Geometry check sheet. Reference: the model listing, model coordinates, mm. A direction names the side the tool comes from. Round coordinates to 2 decimals unless told otherwise and drop trailing zeros. Order: outer loops, then holes, each group sorted by start corner. A loop starts at its lowest first (then second) coordinate and runs counter-clockwise, first axis right, second up. Notation, with made-up numbers: (-20.75, 57.25) -> (34.25, 57.25) arc R13 cw to (34.25, 73.25) -> close; hole circle Ø8 at (2, 12.25). An arc over 180 degrees is marked (long way). Answer as a JSON object with one key per item and string values. Group by question number.
from build123d import *

# Parameters (mm, degrees)
ESBO_O1_R                = 3.05
RESSALTO_EXTRUS_O1_DEPTH = 3
ESBO_O2_W                = 22
ESBO_O2_H                = 82.35
RESSALTO_EXTRUS_O2_DEPTH = 3
RESSALTO_EXTRUS_O3_START = 3
RESSALTO_EXTRUS_O3_DEPTH = 3
ESBO_O6_W                = 85.35
ESBO_O6_H                = 6
RESSALTO_EXTRUS_O5_DEPTH = 3
ESBO_O7_R                = 2.75
RESSALTO_EXTRUS_O6_DEPTH = 0.6


with BuildPart() as part:
    # Esboço1 → Ressalto-extrusão1 (new body)
    with BuildSketch(Plane.XY):
        with BuildLine():
            Line((11, -1.428145739), (11, 25.071854261))
            Line((11, 25.071854261), (-11, 25.071854261))
            Line((-11, 25.071854261), (-11, -1.428145739))
            ThreePointArc((-11, -1.428145739), (0, -12.428145739), (11, -1.428145739))
        make_face()
        with Locations((0, -1.428145739)):
            Circle(ESBO_O1_R, mode=Mode.SUBTRACT)
    extrude(amount=-RESSALTO_EXTRUS_O1_DEPTH)

    # Esboço2 → Ressalto-extrusão2 (add)
    with BuildSketch(Plane(origin=(0, 25.071854261, 0), x_dir=(1, 0, 0), z_dir=(0, 1, 0))):
        with Locations((0, -38.175)):
            Rectangle(ESBO_O2_W, ESBO_O2_H)
    extrude(amount=RESSALTO_EXTRUS_O2_DEPTH)

    # Esboço3 → Ressalto-extrusão3 (add)
    with BuildSketch(Plane.XY.offset(79.35).offset(RESSALTO_EXTRUS_O3_START)):
        with BuildLine():
            Line((11, 28.071854261), (-11, 28.071854261))
            Line((-11, 28.071854261), (-11, -1.428145739))
            ThreePointArc((-11, -1.428145739), (0, -12.428145739), (11, -1.428145739))
            Line((11, -1.428145739), (11, 28.071854261))
        make_face()
    extrude(amount=-RESSALTO_EXTRUS_O3_DEPTH)

    # Esboço6 → Ressalto-extrusão5 (add)
    with BuildSketch(Plane(origin=(11, 0, 0), x_dir=(0, 0, -1), z_dir=(1, 0, 0))):
        with Locations((-39.675, 25.071854261)):
            Rectangle(ESBO_O6_W, ESBO_O6_H)
    ressalto_extrus_o5 = extrude(amount=-RESSALTO_EXTRUS_O5_DEPTH)

    # Espelhar1: Ressalto-extrusão5 across plane
    add(ressalto_extrus_o5.mirror(Plane(origin=(0, 0, 0), x_dir=(0, 0, 1), z_dir=(1, 0, 0))))

    # Esboço7 → Ressalto-extrusão6 (add)
    with BuildSketch(Plane(origin=(0, 0, 79.35), x_dir=(-1, 0, 0), z_dir=(0, 0, -1))):
        with Locations(Location((0, -1.428145739, 0), (0, 0, 180))):
            Circle(ESBO_O7_R)
    extrude(amount=RESSALTO_EXTRUS_O6_DEPTH)


solid = part.part
Item 1: Sectioned sample at B-B, the plane y = 11. Enter the section's corners in (x, z).
Item 2: Thickness scan on L1, parallel to Z at x = 7.5, y = 20; L2, parallel to Y at x = 0, z = -2.1; L3, parallel to Y at x = 8.5, z = 54.5. Record the ranges inside material, lowest first.
Item 3: Mould release check, pull along Y, two halves, no side actions. Record for faces 1 (the flat face through (-10, 22.072, 40)), 2 (the flat face through (0, 28.072, 40)), 3 (the flat face through (0, 7, 79.35)), 4 (the flat face through (-8, 24, 40)): pulls with the +Y half, pulls with the -Y half, needs draft (parallel to the pull), parting line crosses it, or undercut.
Item 4: Depth check by flat-ended pin: pin 1 Ø3.5 at (x, z) = (-10, 49.5) entering from -Y. Enter the tip coordinate at first touch or a pass-through.
Item 5: Sectioned sample at C-C, the plane z = 55.5. Enter the section's corners in (x, y).
Item 6: Sectioned sample at A-A, the plane x = 0. Enter the section's corners in (y, z).
Item 7: Sectioned sample at D-D, the plane y = 24. Enter the section's corners in (x, z), then the cut area to 3 significant figures.
Item 8: Set-up check for faces 5 (the flat face through (0, -1, 78.75)), 6 (the cylindrical face through (-0.397, 1.596, -1.479)), 7 (the flat face through (0, 8, -3)), 8 (the flat face through (8, 24, 40)), 9 (the flat face through (10, 22.072, 40)): record each of +Z, -Z, +X, -X, +Y, -Y from which the full face is reachable in a straight line by a thin tool's end or side.
Result:
{
 "1": {"outline": "(-11, -3) -> (11, -3) -> (11, 0) -> (-11, 0) -> close; (-11, 79.35) -> (11, 79.35) -> (11, 82.35) -> (-11, 82.35) -> close"},
 "2": {"L1": "z = -3 to 0, 79.35 to 82.35", "L2": "y = -12.43 to -4.48, 1.62 to 28.07", "L3": "y = 22.07 to 28.07"},
 "3": {"face 1": "pulls with the -Y half", "face 2": "pulls with the +Y half", "face 3": "undercut", "face 4": "needs draft"},
 "4": {"pin 1": "stops at y = 22.07"},
 "5": {"outline": "(-11, 22.07) -> (-8, 22.07) -> (-8, 25.07) -> (8, 25.07) -> (8, 22.07) -> (11, 22.07) -> (11, 28.07) -> (-11, 28.07) -> close"},
 "6": {"outline": "(-12.43, -3) -> (-4.48, -3) -> (-4.48, 0) -> (-12.43, 0) -> close; (-12.43, 79.35) -> (-4.18, 79.35) -> (-4.18, 78.75) -> (1.32, 78.75) -> (1.32, 79.35) -> (25.07, 79.35) -> (25.07, 0) -> (1.62, 0) -> (1.62, -3) -> (28.07, -3) -> (28.07, 82.35) -> (-12.43, 82.35) -> close"},
 "7": {"outline": "(-11, -3) -> (11, -3) -> (11, 82.35) -> (-11, 82.35) -> close; hole (-8, 0) -> (8, 0) -> (8, 79.35) -> (-8, 79.35) -> close", "area": "608 mm2"},
 "8": {"face 5": "-Z, +X, -X, -Y", "face 6": "-Z", "face 7": "-Z, +X, -X, +Y, -Y", "face 8": "-Y", "face 9": "+X, -X, -Y"}
}
